Part model, mm, in its own coordinate system. A direction names the side the tool comes from. Coordinates: 2 decimals unless noted, no trailing zeros. Loops run counter-clockwise (first coordinate to the right, second up) from the corner with the lowest first, then second, coordinate; pieces in that order, holes last. Notation, with made-up numbers: M 35,1 L 91,1 A24 cw 91,27 Z; hole C 56.5,76.5 d5. An arc over 180 degrees is marked long. Use a Markdown table: item, result. Add a question column.
1) Band-saw the part on B-B (x = 0). List the corners of the cut face in (y, z), plus the area to 3 significant figures.
2) Tool access for faces 4 (the flat face through (-9, 10, 0)), 5 (the flat face through (-40.9, 18, 1)), 6 (the flat face through (0, 5.11, 1)): list every direction of +Z, -Z, +X, -X, +Y, -Y with a clear straight run to the whole face (end or side of a thin tool).
3) Band-saw the part on C-C (x = -42). List the corners of the cut face in (y, z), plus the area to 3 significant figures.
4) Band-saw the part on D-D (z = 1.6). State how many separate pieces and enclosed holes the cut face has, plus the area to 3 significant figures.
5) Pull direction Y, two halves, no side cores. Call faces 1 (the flat face through (-25.7, -12, 1)), 2 (the cylindrical face through (-41.983, 14.454, 0.986)), 3 (the flat face through (-43.03, 28.21, 0.99)): released by +Y, released by -Y, zero draft, split by the parting line, or undercut.
6) Band-saw the part on A-A (y = -2). List the corners of the cut face in (x, z), plus the area to 3 significant figures.
7) Pin check, flat tips, straight feed: pin 1 Ø2.5 at (x, y) = (26.8, 9.51) entering from -Z; pin 2 Ø0.6 at (x, z) = (41.5, 1) entering from +Y. Stop position of each tip, or through.
8) Wall check: probe 1 along X at (y, z) = (-17.5, 1.25); probe 2 along Y at (x, z) = (32, 1.2); probe 3 along X at (y, z) = (9, 0.85). Give the ranges that are in metal, low to high. Write a range as from..to.
from build123d import *

# Parameters (mm, degrees)
SKETCH_3_R      = 2.2
SKETCH_3_R_2    = 1.5
EXTRUDE_1_DEPTH = 2


with BuildPart() as part:
    # 草图3 → 凸台-拉伸1 (new body)
    with BuildSketch(Plane.XY):
        with BuildLine():
            Line((-41, -23.990216685), (-42, -23.990216685))
            Line((-42, -23.990216685), (-44, -23.990216685))
            Line((-44, -23.990216685), (-45, -23.990216685))
            Line((-45, -23.990216685), (-45, 5.009783315))
            Line((-45, 5.009783315), (-45, 15.009783315))
            Line((-45, 15.009783315), (-45, 26.463053661))
            Line((-45, 26.463053661), (-41, 30.009783315))
            ThreePointArc((-41, 30.009783315), (-34.419700625, 29.918417102), (-28.474223323, 27.097072158))
            ThreePointArc((-28.474223323, 27.097072158), (-27.224142294, 25.7867036), (-25.913822519, 24.536571436))
            ThreePointArc((-25.913822519, 24.536571436), (-15.930575575, 14.55280442), (-1.811764604, 14.552436852))
            ThreePointArc((-1.811764604, 14.552436852), (0, 14.509783471), (1.811764604, 14.552436852))
            ThreePointArc((1.811764604, 14.552436852), (15.930575575, 14.55280442), (25.913822519, 24.536571436))
            ThreePointArc((25.913822519, 24.536571436), (27.224142294, 25.7867036), (28.474223323, 27.097072158))
            ThreePointArc((28.474223323, 27.097072158), (34.419700625, 29.918417102), (41, 30.009783315))
            Line((41, 30.009783315), (45, 26.463053661))
            Line((45, 26.463053661), (45, 15.009783315))
            Line((45, 15.009783315), (45, -23.990216685))
            Line((45, -23.990216685), (41, -23.990216685))
            Line((41, -23.990216685), (25.7, -23.990216685))
            Line((25.7, -23.990216685), (25.7, -19.890216685))
            Line((25.7, -19.890216685), (25.7, -18.890216685))
            Line((25.7, -18.890216685), (25.7, 0.109783315))
            ThreePointArc((25.7, 0.109783315), (24.235533906, 3.645317221), (20.7, 5.109783315))
            Line((20.7, 5.109783315), (-20.7, 5.109783315))
            ThreePointArc((-20.7, 5.109783315), (-24.235533906, 3.645317221), (-25.7, 0.109783315))
            Line((-25.7, 0.109783315), (-25.7, -18.890216685))
            Line((-25.7, -18.890216685), (-25.7, -19.890216685))
            Line((-25.7, -19.890216685), (-25.7, -23.990216685))
            Line((-25.7, -23.990216685), (-41, -23.990216685))
        make_face()
        with Locations((0, 10.509783315)):
            Circle(SKETCH_3_R, mode=Mode.SUBTRACT)
        with Locations((-30.0520382, 22.957745114)):
            Circle(SKETCH_3_R, mode=Mode.SUBTRACT)
        with Locations((30.0520382, 22.957745114)):
            Circle(SKETCH_3_R, mode=Mode.SUBTRACT)
        with Locations((-26.8, 9.509783315)):
            Circle(SKETCH_3_R_2, mode=Mode.SUBTRACT)
        with Locations(Location((26.8, 9.509783315, 0), (0, 0, 180))):
            Circle(SKETCH_3_R_2, mode=Mode.SUBTRACT)
        with Locations((42, 10.009783315)):
            Circle(SKETCH_3_R_2, mode=Mode.SUBTRACT)
        with Locations(Location((-42, 10.009783315, 0), (0, 0, 180))):
            Circle(SKETCH_3_R_2, mode=Mode.SUBTRACT)
        with BuildLine():
            Line((-37.1, -22.090216685), (-29.9, -22.090216685))
            Line((-29.9, -22.090216685), (-29.9, -19.890216685))
            Line((-29.9, -19.890216685), (-37.1, -19.890216685))
            ThreePointArc((-37.1, -19.890216685), (-37.555634919, -20.990216685), (-37.1, -22.090216685))
        make_face(mode=Mode.SUBTRACT)
        with BuildLine():
            Line((29.9, -22.090216685), (29.9, -19.890216685))
            Line((29.9, -19.890216685), (37.1, -19.890216685))
            ThreePointArc((37.1, -19.890216685), (37.555634919, -20.990216685), (37.1, -22.090216685))
            Line((37.1, -22.090216685), (29.9, -22.090216685))
        make_face(mode=Mode.SUBTRACT)
        with BuildLine():
            Line((-43.1, 5.109783315), (-43.1, -0.090216685))
            Line((-43.1, -0.090216685), (-40.9, -0.090216685))
            Line((-40.9, -0.090216685), (-40.9, 5.109783315))
            ThreePointArc((-40.9, 5.109783315), (-42, 5.565418233), (-43.1, 5.109783315))
        make_face(mode=Mode.SUBTRACT)
        with BuildLine():
            Line((-43.1, 20.109783315), (-40.9, 20.109783315))
            Line((-40.9, 20.109783315), (-40.9, 14.909783315))
            ThreePointArc((-40.9, 14.909783315), (-42, 14.454148396), (-43.1, 14.909783315))
            Line((-43.1, 14.909783315), (-43.1, 20.109783315))
        make_face(mode=Mode.SUBTRACT)
        with BuildLine():
            Line((40.9, 20.109783315), (40.9, 14.909783315))
            ThreePointArc((40.9, 14.909783315), (42, 14.454148396), (43.1, 14.909783315))
            Line((43.1, 14.909783315), (43.1, 20.109783315))
            Line((43.1, 20.109783315), (40.9, 20.109783315))
        make_face(mode=Mode.SUBTRACT)
        with BuildLine():
            Line((40.9, 5.109783315), (40.9, -0.090216685))
            Line((40.9, -0.090216685), (43.1, -0.090216685))
            Line((43.1, -0.090216685), (43.1, 5.109783315))
            ThreePointArc((43.1, 5.109783315), (42, 5.565418233), (40.9, 5.109783315))
        make_face(mode=Mode.SUBTRACT)
    extrude(amount=EXTRUDE_1_DEPTH)


solid = part.part
Entries:
| question | item | result |
|---|---|---|
| 1 | outline | M 5.11,0 L 8.31,0 L 8.31,2 L 5.11,2 Z; M 12.71,0 L 14.51,0 L 14.51,2 L 12.71,2 Z |
| 1 | area | 10.0 mm2 |
| 2 | face 4 | -Z, +X, -X, +Y, -Y |
| 2 | face 5 | +Z, -Z |
| 2 | face 6 | +Z, -Z, -Y |
| 3 | outline | M -23.99,0 L -0.09,0 L -0.09,2 L -23.99,2 Z; M 5.57,0 L 8.51,0 L 8.51,2 L 5.57,2 Z; M 11.51,0 L 14.45,0 L 14.45,2 L 11.51,2 Z; M 20.11,0 L 29.12,0 L 29.12,2 L 20.11,2 Z |
| 3 | area | 77.6 mm2 |
| 4 | separate pieces | 1 |
| 4 | enclosed holes | 13 |
| 4 | area | 2,420 mm2 |
| 5 | face 1 | zero draft |
| 5 | face 2 | undercut |
| 5 | face 3 | released by +Y |
| 6 | outline | M -45,0 L -25.7,0 L -25.7,2 L -45,2 Z; M 25.7,0 L 45,0 L 45,2 L 25.7,2 Z |
| 6 | area | 77.2 mm2 |
| 7 | pin 1 | through |
| 7 | pin 2 | y = 29.83 |
| 8 | probe 1 | -45..-25.7, 25.7..45 |
| 8 | probe 2 | -23.99..-22.09, -19.89..21.94, 23.98..29.14 |
| 8 | probe 3 | -45..-43.11, -40.89..-28.21, -25.39..-1.6, 1.6..25.39, 28.21..40.89, 43.11..45 |
